Input: part model. Units: mm. Frame: model coordinates. A direction names the side the tool comes from. Round coordinates to 2 decimals unless told otherwise and drop trailing zeros. Loops run counter-clockwise (first coordinate to the right, second up) from the corner with the lowest first, then second, coordinate; pieces in that order, holes last. Notation, with made-up numbers: (-5.5, 35.5) - (-0.5, 35.5) arc R28 cw to (-0.5, 57.5) - close; hole circle Ø9 at (-17, -35.5). An arc over 180 degrees is marked (long way). One line per question, with ' | ' between items. Start each with the question number.
Item 1: First-contact query: pin 1 (2.5 mm diameter, centred on y = 32.8, z = 25.41, fed in from +X); pin 2 (0.8 mm diameter, centred on x = 0.5, z = -37.5, fed in from -Y); pin 3 (0.8 mm diameter, centred on x = 1, y = 13.5, fed in from +Z); pin 4 (0.8 mm diameter, centred on x = 0.5, y = 5.5, fed in from +Z). Flat tips, straight axial feed; report the tip coordinate or a pass-through.
Item 2: Draft query along Y for faces 3 (the face through (0.8, 22.6, -51.6)), 4 (the face through (0, 20, 23)), 5 (the face through (0.79, 7.59, -46)), 6 (the face through (0.811, 33.862, 39.573)). Return one class per face: pulls with the +Y half, pulls with the -Y half, needs draft (parallel to the pull), parting line crosses it, or undercut.
Item 3: Set-up query: faces 1 (the face through (1.6, 20, 23)), 2 (the face through (0.81, 33.67, 62.29)). Return all of +Z, -Z, +X, -X, +Y, -Y with unobstructed straight access to the full face (end or side cutting, diameter ignored); none if empty.
Item 4: Section B-B, the plane z = 33.5. Give the number of separate pieces and of enclosed holes in the cut face, plus the area to 3 significant figures.
Item 5: Section D-D, the plane y = 48. Return loops of the section in (x, z), plus the area to 3 significant figures.
Item 6: Section A-A, the plane z = 14. Return loops of the section in (x, y).
Item 7: Material intervals for line 1 along Y through (x, z) = (1.1, 36); line 2 along Y through (x, z) = (1.55, 14); line 3 along Z through (x, y) = (0.95, 34), sorted ascending.
```python
from build123d import *

# Parameters (mm, degrees)
SKETCH_215_W           = 23.879073069
SKETCH_215_H           = 2
SKETCH_215_W_2         = 13.873866224
SKETCH_215_H_2         = 3.944574251
EXTRUDE_1_DEPTH        = 1.6
SKETCH_2_W             = 8
SKETCH_2_H             = 1.6
EXTRUDE_3744_DEPTH     = 1.6
SKETCH_3858_R          = 1.575
SKETCH_3858_RX         = 4.079397779
SKETCH_3858_RY         = 3.125
CUT_EXTRUDE_4259_DEPTH = 111.010448945
CUT_EXTRUDE_4725_DEPTH = 111.010449082
USB_C_DEPTH            = 111.010449082


with BuildPart() as part:
    # Sketch 215 → 凸台-拉伸1 (new body)
    with BuildSketch(Plane(origin=(0, 0, 0), x_dir=(0, 0, -1), z_dir=(1, 0, 0))):
        with BuildLine():
            Line((-95.202576637, 16.678130112), (-96.66172395, 0))
            Line((-96.66172395, 0), (-44.182229478, 0))
            ThreePointArc((-44.182229478, 0), (-41.932229478, 2.25), (-39.682229478, 0))
            Line((-39.682229478, 0), (-23.132229478, 0))
            ThreePointArc((-23.132229478, 0), (-20.882229478, 2.25), (-18.632229478, 0))
            Line((-18.632229478, 0), (38.58827605, 0))
            Line((38.58827605, 0), (38.58827605, 5.363667343))
            Line((38.58827605, 5.363667343), (53.613979238, 9.877821069))
            Line((53.613979238, 9.877821069), (53.613979238, 20.082386187))
            Line((53.613979238, 20.082386187), (49.47062371, 25.265958003))
            ThreePointArc((49.47062371, 25.265958003), (48.834122057, 24.360802519), (48.136507156, 23.501864655))
            Line((48.136507156, 23.501864655), (49.140587437, 22.184380908))
            Line((49.140587437, 22.184380908), (47.555615421, 20.806751165))
            Line((47.555615421, 20.806751165), (46.571594176, 21.938874033))
            Line((46.571594176, 21.938874033), (44.304779315, 24.546859335))
            ThreePointArc((44.304779315, 24.546859335), (45.901319607, 26.216879129), (47.163951689, 28.151735001))
            Line((47.163951689, 28.151735001), (38.58827605, 38.88038965))
            Line((38.58827605, 38.88038965), (37.693344157, 40))
            Line((37.693344157, 40), (-18.632229478, 40))
            ThreePointArc((-18.632229478, 40), (-20.882229478, 37.75), (-23.132229478, 40))
            Line((-23.132229478, 40), (-39.682229478, 40))
            ThreePointArc((-39.682229478, 40), (-41.932229478, 37.75), (-44.182229478, 40))
            Line((-44.182229478, 40), (-87.664190365, 40))
            ThreePointArc((-87.664190365, 40), (-91.717731611, 38.423664021), (-93.641358554, 34.522934456))
            Line((-93.641358554, 34.522934456), (-94.87665585, 20.403421746))
            ThreePointArc((-94.87665585, 20.403421746), (-92.775563539, 19.482408503), (-90.560913042, 18.883929203))
            Line((-90.560913042, 18.883929203), (-91.219638908, 15.446476624))
            Line((-91.219638908, 15.446476624), (-91.483129255, 14.071495593))
            Line((-91.483129255, 14.071495593), (-93.545600802, 14.466731113))
            Line((-93.545600802, 14.466731113), (-93.260074318, 15.956704104))
            ThreePointArc((-93.260074318, 15.956704104), (-94.241224457, 16.290763242), (-95.202576637, 16.678130112))
        make_face()
        with Locations((-32.321766012, 13.338077)):
            Rectangle(SKETCH_215_W, SKETCH_215_H, mode=Mode.SUBTRACT)
        with Locations((-32.321766012, 17.395875517)):
            Rectangle(SKETCH_215_W, SKETCH_215_H, mode=Mode.SUBTRACT)
        with Locations((-12.198657062, 12.527713279)):
            Rectangle(SKETCH_215_W_2, SKETCH_215_H_2, mode=Mode.SUBTRACT)
        with BuildLine():
            Line((-87.309268426, 30.113751112), (-88.369968079, 30.317015094))
            Line((-88.369968079, 30.317015094), (-89.430667732, 30.520279076))
            Line((-89.430667732, 30.520279076), (-89.890653352, 33.675403991))
            ThreePointArc((-89.890653352, 33.675403991), (-87.826914488, 36.244108032), (-85.414190365, 34))
            ThreePointArc((-85.414190365, 34), (-85.490811978, 33.417826153), (-85.715458265, 32.875303062))
            Line((-85.715458265, 32.875303062), (-87.309268426, 30.113751112))
        make_face(mode=Mode.SUBTRACT)
        with BuildLine():
            ThreePointArc((34.968023431, 32.04870964), (34.612244182, 35.698184303), (38.176585209, 34.837534989))
            Line((38.176585209, 34.837534989), (39.363457628, 31.878188125))
            Line((39.363457628, 31.878188125), (38.548329162, 31.169692829))
            Line((38.548329162, 31.169692829), (37.733200697, 30.461197532))
            Line((37.733200697, 30.461197532), (34.968023431, 32.04870964))
        make_face(mode=Mode.SUBTRACT)
    extrude(amount=EXTRUDE_1_DEPTH)

    # 草图2 → Extrude 3744 (add)
    with BuildSketch(Plane(origin=(0, 0, 0), x_dir=(0, 0, -1), z_dir=(1, 0, 0))):
        with Locations((31.58827605, -0.8)):
            Rectangle(SKETCH_2_W, SKETCH_2_H)
        with BuildLine():
            Line((-83.862737476, 52.5), (-85.358986401, 42))
            ThreePointArc((-85.358986401, 42), (-86.138250874, 40.569690448), (-87.664190365, 40))
            Line((-87.664190365, 40), (-65.306655843, 40))
            Line((-65.306655843, 40), (-57.306655843, 40))
            Line((-57.306655843, 40), (-57.306655843, 41.6))
            Line((-57.306655843, 41.6), (-65.306655843, 41.6))
            Line((-65.306655843, 41.6), (-75.139107316, 52.5))
            Line((-75.139107316, 52.5), (-83.862737476, 52.5))
        make_face()
        with Locations((1.58827605, -0.8)):
            Rectangle(SKETCH_2_W, SKETCH_2_H)
        with Locations((-58.41172395, -0.8)):
            Rectangle(SKETCH_2_W, SKETCH_2_H)
        with Locations((-88.41172395, -0.8)):
            Rectangle(SKETCH_2_W, SKETCH_2_H)
        with Locations((28.693344157, 40.8)):
            Rectangle(SKETCH_2_W, SKETCH_2_H)
        with Locations((-1.306655843, 40.8)):
            Rectangle(SKETCH_2_W, SKETCH_2_H)
        with Locations((-31.306655843, 40.8)):
            Rectangle(SKETCH_2_W, SKETCH_2_H)
    extrude(amount=EXTRUDE_3744_DEPTH)

    # Sketch 3858 → Cut-Extrude 4259 (cut, through all)
    with BuildSketch(Plane(origin=(1.6, 0, 0), x_dir=(0, 0, -1), z_dir=(1, 0, 0))):
        with Locations((-38.41172395, 32.797244765)):
            Circle(SKETCH_3858_R)
        with Locations((-25.41172395, 32.797244765)):
            Circle(SKETCH_3858_R)
        with Locations(Location((-31.91172395, 25.645875517), (0, 0, 90))):
            Ellipse(SKETCH_3858_RX, SKETCH_3858_RY)
    extrude(amount=-CUT_EXTRUDE_4259_DEPTH, mode=Mode.SUBTRACT)

    # 草图3 → Cut-Extrude 4725 (cut, through all)
    with BuildSketch(Plane(origin=(1.6, 0, 0), x_dir=(0, 0, -1), z_dir=(1, 0, 0))):
        with BuildLine():
            Line((-71.837081834, 30.223280517), (-73.468745408, 11.573280517))
            ThreePointArc((-73.468745408, 11.573280517), (-76.908383058, 8.687081834), (-79.794581741, 12.126719483))
            Line((-79.794581741, 12.126719483), (-78.162918166, 30.776719483))
            ThreePointArc((-78.162918166, 30.776719483), (-74.723280517, 33.662918166), (-71.837081834, 30.223280517))
        make_face()
        with BuildLine():
            Line((17.026747393, 32.354992688), (28.419615873, 16.52930004))
            ThreePointArc((28.419615873, 16.52930004), (27.697861168, 12.097559959), (23.266121087, 12.819314663))
            Line((23.266121087, 12.819314663), (11.873252607, 28.645007312))
            ThreePointArc((11.873252607, 28.645007312), (12.595007312, 33.076747393), (17.026747393, 32.354992688))
        make_face()
        with BuildLine():
            Line((2.026747393, 32.354992688), (13.419615873, 16.52930004))
            ThreePointArc((13.419615873, 16.52930004), (12.697861168, 12.097559959), (8.266121087, 12.819314663))
            Line((8.266121087, 12.819314663), (-3.126747393, 28.645007312))
            ThreePointArc((-3.126747393, 28.645007312), (-2.404992688, 33.076747393), (2.026747393, 32.354992688))
        make_face()
        with BuildLine():
            Line((-59.337081834, 30.223280517), (-60.968745408, 11.573280517))
            ThreePointArc((-60.968745408, 11.573280517), (-64.408383058, 8.687081834), (-67.294581741, 12.126719483))
            Line((-67.294581741, 12.126719483), (-65.662918166, 30.776719483))
            ThreePointArc((-65.662918166, 30.776719483), (-62.223280517, 33.662918166), (-59.337081834, 30.223280517))
        make_face()
    extrude(amount=-CUT_EXTRUDE_4725_DEPTH, mode=Mode.SUBTRACT)

    # Sketch1 → USB-C供电接口 (cut, through all)
    with BuildSketch(Plane(origin=(0, 0, 0), x_dir=(0, 0, -1), z_dir=(1, 0, 0))):
        with BuildLine():
            Line((-76.136302547, 6.588077), (-67.386302547, 6.588077))
            ThreePointArc((-67.386302547, 6.588077), (-67.032749156, 6.441630391), (-66.886302547, 6.088077))
            Line((-66.886302547, 6.088077), (-66.886302547, 4.088077))
            ThreePointArc((-66.886302547, 4.088077), (-67.032749156, 3.734523609), (-67.386302547, 3.588077))
            Line((-67.386302547, 3.588077), (-76.136302547, 3.588077))
            ThreePointArc((-76.136302547, 3.588077), (-76.489855937, 3.734523609), (-76.636302547, 4.088077))
            Line((-76.636302547, 4.088077), (-76.636302547, 6.088077))
            ThreePointArc((-76.636302547, 6.088077), (-76.489855937, 6.441630391), (-76.136302547, 6.588077))
        make_face()
        with BuildLine():
            Line((-79.011302547, 4.063077), (-80.261302547, 4.063077))
            ThreePointArc((-80.261302547, 4.063077), (-81.286302547, 5.088077), (-80.261302547, 6.113077))
            Line((-80.261302547, 6.113077), (-79.011302547, 6.113077))
            ThreePointArc((-79.011302547, 6.113077), (-77.986302547, 5.088077), (-79.011302547, 4.063077))
        make_face()
        with BuildLine():
            Line((-64.511302547, 4.063077), (-63.261302547, 4.063077))
            ThreePointArc((-63.261302547, 4.063077), (-62.236302547, 5.088077), (-63.261302547, 6.113077))
            Line((-63.261302547, 6.113077), (-64.511302547, 6.113077))
            ThreePointArc((-64.511302547, 6.113077), (-65.536302547, 5.088077), (-64.511302547, 4.063077))
        make_face()
    extrude(amount=USB_C_DEPTH, mode=Mode.SUBTRACT)


solid = part.part
```
Return value:
1) pin 1: through | pin 2: y = 0 | pin 3: z = 95.52 | pin 4: z = 96.22
2) face 3: pulls with the +Y half | face 4: needs draft | face 5: pulls with the -Y half | face 6: undercut
3) face 1: +Z, -Z, +X, +Y, -Y | face 2: +X, -X
4) separate pieces: 4 | enclosed holes: 0 | area: 48.9 mm2
5) outline: (0, 71.08) - (1.6, 71.08) - (1.6, 84.5) - (0, 84.5) - close | area: 21.5 mm2
6) outline: (0, 0) - (1.6, 0) - (1.6, 10.56) - (0, 10.56) - close; (0, 14.5) - (1.6, 14.5) - (1.6, 40) - (0, 40) - close
7) line 1: 0 to 12.34, 14.34 to 16.4, 18.4 to 40 | line 2: 0 to 10.56, 14.5 to 40 | line 3: -42.49 to -38.51, -33.84 to 24.39, 26.43 to 37.39, 39.43 to 85.41, 89.91 to 93.69
